Autodesk Inventor part; units mm, degrees
ref_plane "YZ Plane" through (0, 0, 0) normal (1, 0, 0) x (0, 1, 0)
ref_plane "XZ Plane" through (0, 0, 0) normal (0, 1, 0) x (-1, 0, 0)
ref_plane "XY Plane" through (0, 0, 0) normal (0, 0, 1) x (1, 0, 0)
sketch "Skizze1" plane through (0, 0, 0) normal (0, 0, 1) x (1, 0, 0)
  line L0 (0, 0) -> (144, 0)
  line L1 (144, 50) -> (0, 50)
  line L2 (72, 50) -> (72, 0) construction
  circle A0 centre (72, 34) radius 4
  line L3 (0, 50) -> (0, 0)
  line L4 (144, 0) -> (144, 50)
  line L5 (0, 20) -> (144, 20) construction
  line L6 (0, 34) -> (144, 34) construction
  circle A1 centre (105, 20) radius 1.5
  circle A2 centre (25, 20) radius 1.5
  circle A3 centre (65, 20) radius 1.5
  dimension "d17" = 8
  dimension "d207" = 50
  dimension "d224" = 144
  dimension "d225" = 20
  dimension "d226" = 34
  dimension "d228" = 3
  dimension "d229" = 3
  dimension "d232" = 3
  dimension "d233" = 7
  dimension "d234" = 40
  dimension "d235" = 40
extrude "Extrusion1" add sketch "Skizze1" along normal blind 30 contours L3 L1 L4 L0 | A1 | A2 | A3
sketch "Skizze7" plane through (0, 0, 0) normal (0, 0, -1) x (-1, 0, 0)
  line L0 (0, 0) -> (-144, 0) construction
  line L1 (-144, 50) -> (0, 50) construction
  line L2 (-144, 0) -> (-144, 50) construction
  line L3 (0, 50) -> (0, 0) construction
  line L4 (-144, 0) -> (-144, 50)
  line L5 (-144, 20) -> (0, 20) construction
  line L6 (0, 0) -> (-144, 0) construction
  line L7 (-72, 0) -> (-72, 50) construction
  point P0 (-79, 20)
  point P1 (-119, 20)
  point P2 (-39, 20)
  dimension "d236" = 7
  dimension "d237" = 20
  dimension "d238" = 40
  dimension "d239" = 40
hole "Bohrung19" at (79, 20, 0) at (119, 20, 0) at (39, 20, 0) direction (0, 0, 1) diameter 2.5 depth 25 tip angle 118
sketch "Skizze8" plane through (0, 0, 0) normal (0, -1, 0) x (1, 0, 0)
  line L0 (144, 0) -> (144, 30) construction
  line L1 (0, 30) -> (144, 30) construction
  line L2 (0, 0) -> (144, 0) construction
  line L3 (144, 0) -> (144, 30) construction
  line L4 (0, 30) -> (144, 30) construction
  line L5 (0, 0) -> (0, 30) construction
  line L6 (144, 17) -> (0, 17) construction
  line L7 (25, 30) -> (25, 0) construction
  line L8 (0, 0) -> (144, 0) construction
  point P0 (25, 17)
  point P1 (65, 17)
  point P2 (105, 17)
  dimension "d247" = 17
  dimension "d248" = 25
  dimension "d249" = 40
  dimension "d250" = 40
hole "Bohrung20" at (25, 0, 17) at (65, 0, 17) at (105, 0, 17) direction (0, 1, 0) diameter 2.5 depth 30 tip angle 118
sketch "Skizze9" plane through (144, 0, 0) normal (1, 0, 0) x (0, 0, -1)
  line L0 (0, 0) -> (0, 50) construction
  line L1 (0, 50) -> (-30, 50) construction
  line L2 (-30, 0) -> (-30, 50) construction
  line L3 (0, 0) -> (-30, 0) construction
  line L4 (0, 0) -> (-30, 0) construction
  line L5 (-13, 0) -> (-13, 50) construction
  point P0 (-13, 14)
  point P1 (-13, 39)
  dimension "d258" = 13
  dimension "d259" = 14
  dimension "d261" = 25
hole "Bohrung21" at (144, 14, 13) at (144, 39, 13) direction (-1, 0, 0) diameter 2.5 depth 30 tip angle 118
properties part number "licht_150_support_right"
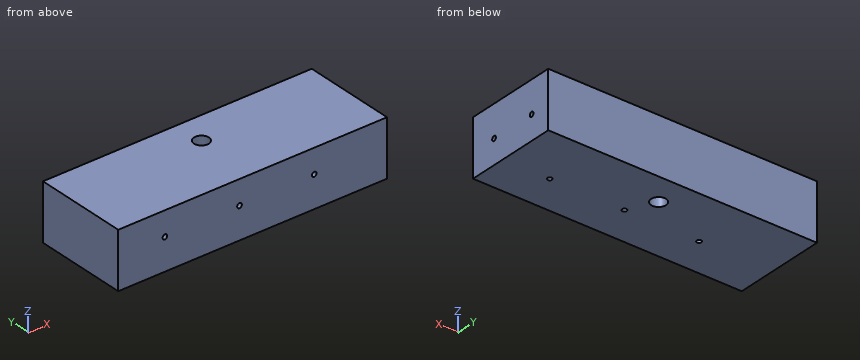
For this review, take the finished solid that the model builds, in its own axes (mm). Round coordinates to 2 decimals unless told otherwise and drop trailing zeros. Order: outer loops, then holes, each group sorted by start corner. A loop starts at its lowest first (then second) coordinate and runs counter-clockwise, first axis right, second up.
Q1. Insertion check: P1, Ø6.5, axis at x = 72, y = 34, coming from the +Z side; P2, Ø3, axis at x = 89.5, z = 16, coming from the -Y side. Each pin has a flat end and moves straight along its axis. Give the tip position at first contact, or say it passes through.
Findings below:
P1: passes through
P2: stops at y = 0
Q2. We need section A-A, the plane y = 34. Give the boundary of the cut face in (x, z).
Findings below:
outline: (0, 0) - (68, 0) - (68, 30) - (0, 30) - close; (76, 0) - (144, 0) - (144, 30) - (76, 30) - close
Q3. Wall thickness on line 1 (X direction, y = 20, z = 8.5); line 2 (Y direction, x = 125.5, z = 13); line 3 (X direction, y = 23.5, z = 17): over which ranges is each line inside the solid? List them lowest first.
Findings below:
line 1: x = 0 to 37.75, 40.25 to 77.75, 80.25 to 117.75, 120.25 to 144
line 2: y = 0 to 12.75, 15.25 to 37.75, 40.25 to 50
line 3: x = 0 to 23.75, 26.25 to 63.75, 66.25 to 103.75, 106.25 to 144
Q4. We need section B-B, the plane x = 72. Give the boundary of the cut face in (y, z).
Findings below:
outline: (0, 0) - (30, 0) - (30, 30) - (0, 30) - close; (38, 0) - (50, 0) - (50, 30) - (38, 30) - close
